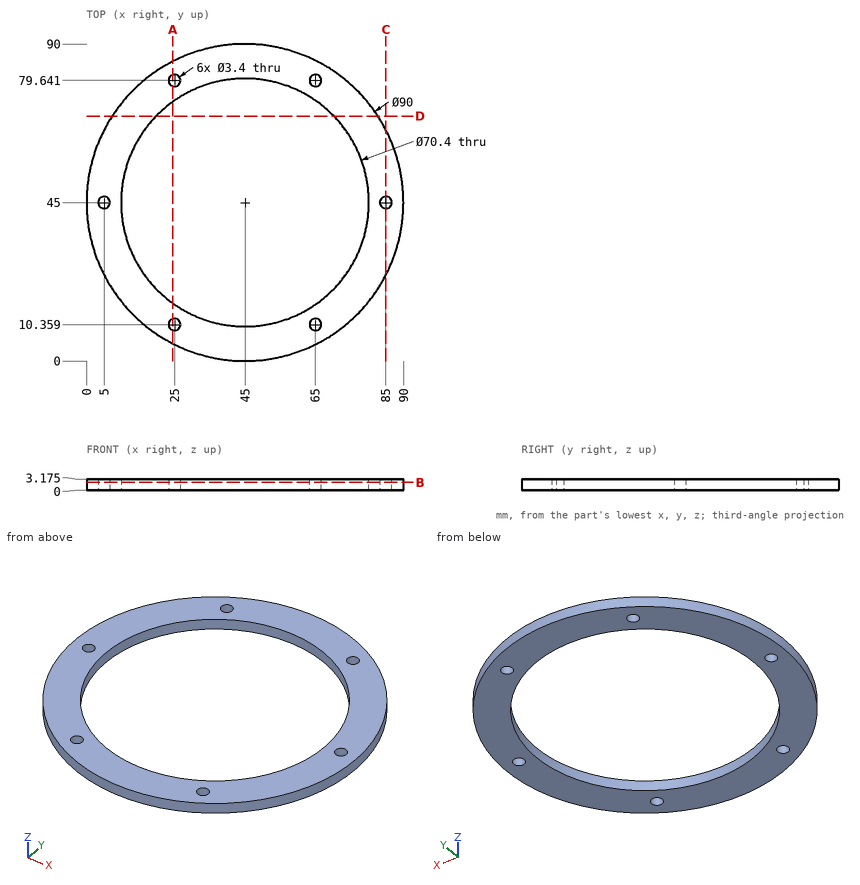
Source: three-view drawing plus pictorial views. Frame: mm from the lowest corner of the part. Round coordinates to 2 decimals unless told otherwise and drop trailing zeros. Order: outer loops, then holes, each group sorted by start corner. A loop starts at its lowest first (then second) coordinate and runs counter-clockwise, first axis right, second up. Notation, with made-up numbers: (18.25, -5.75) -> (70.25, -5.75) arc R31 cw to (70.25, 21.25) -> close; hole circle Ø2 at (29, 60.25). An arc over 180 degrees is marked (long way). Use one line per item in the form item = value. Start each with the question number.
1. Cut plane A-A (x = 24.5). Return the cut outline in (y, z) (1 decimal), then the cut area to 3 significant figures.
2. Line query: probe 1 along Y at (x, z) = (25, 1.25); probe 2 along Y at (x, z) = (44, 0.75); probe 3 along X at (y, z) = (67, 0.4). Output: solid intervals per line, ascending.
3. Pin query (flat end, axial travel): pin 1 Ø1 at (y, z) = (52.5, 1.5) entering from -X; pin 2 Ø1 at (x, z) = (31, 1.5) entering from -Y; pin 3 Ø1.5 at (x, z) = (34, 1) entering from +Y. Return the tip coordinate at first contact, or that it passes through.
4. Cut plane C-C (x = 85). Return the cut outline in (y, z) (1 decimal), then the cut area to 3 significant figures.
5. Cut plane D-D (y = 69.5). Return the cut outline in (x, z) (3 decimals).
6. Cut plane B-B (z = 2.25). Return the cut outline in (x, y), then the cut area to 3 significant figures.
Solution:
q1.outline = (4.9, 0) -> (8.7, 0) -> (8.7, 3.2) -> (4.9, 3.2) -> close; (12, 0) -> (16.4, 0) -> (16.4, 3.2) -> (12, 3.2) -> close; (73.6, 0) -> (78, 0) -> (78, 3.2) -> (73.6, 3.2) -> close; (81.3, 0) -> (85.1, 0) -> (85.1, 3.2) -> (81.3, 3.2) -> close
q1.area = 52.0 mm^2
q2.probe_1 = 4.69 to 8.66, 12.06 to 16.03, 73.97 to 77.94, 81.34 to 85.31
q2.probe_2 = 0.01 to 9.81, 80.19 to 89.99
q2.probe_3 = 5.74 to 17.52, 72.48 to 84.26
q3.pin_1 = 0.55
q3.pin_2 = 2.07
q3.pin_3 = 88.82
q4.outline = (24.4, 0) -> (43.3, 0) -> (43.3, 3.2) -> (24.4, 3.2) -> close; (46.7, 0) -> (65.6, 0) -> (65.6, 3.2) -> (46.7, 3.2) -> close
q4.area = 120 mm^2
q5.outline = (7.254, 0) -> (19.726, 0) -> (19.726, 3.175) -> (7.254, 3.175) -> close; (70.274, 0) -> (82.746, 0) -> (82.746, 3.175) -> (70.274, 3.175) -> close
q6.outline = circle Ø90 at (45, 45); hole circle Ø3.4 at (5, 45); hole circle Ø70.4 at (45, 45); hole circle Ø3.4 at (25, 10.36); hole circle Ø3.4 at (25, 79.64); hole circle Ø3.4 at (65, 10.36); hole circle Ø3.4 at (65, 79.64); hole circle Ø3.4 at (85, 45)
q6.area = 2,410 mm^2
